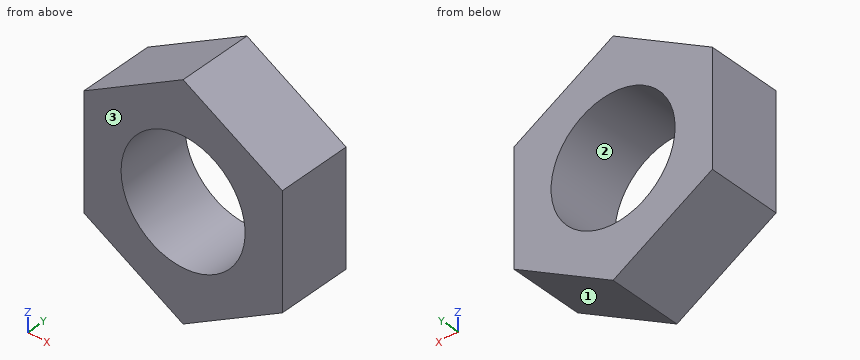
Autodesk Inventor part; units mm, degrees
ref_plane "YZ Plane" through (0, 0, 0) normal (1, 0, 0) x (0, 1, 0)
ref_plane "XZ Plane" through (0, 0, 0) normal (0, 1, 0) x (-1, 0, 0)
ref_plane "XY Plane" through (0, 0, 0) normal (0, 0, 1) x (1, 0, 0)
sketch "Sketch1" plane through (0, 0, 0) normal (0, 1, 0) x (-1, 0, 0)
  line L0 (0, -4.6188) -> (-4, -2.3094)
  line L1 (-4, -2.3094) -> (-4, 2.3094)
  line L2 (-4, 2.3094) -> (0, 4.6188)
  line L3 (0, 4.6188) -> (4, 2.3094)
  line L4 (4, 2.3094) -> (4, -2.3094)
  line L5 (4, -2.3094) -> (0, -4.6188)
  circle A0 centre (0, 0) radius 2.5
  dimension "d0" = 8
  dimension "d1" = 5
extrude "Extrusion1" add sketch "Sketch1" along normal blind 3
thread "Thread1"
properties part number "nut rod"
Could you check a few things on this model? Use its own coordinates, in mm. Face numbers are marked on the shaded views. Coordinates: 2 decimals unless noted, no trailing zeros. Order: outer loops, then holes, each group sorted by start corner. A loop starts at its lowest first (then second) coordinate and runs counter-clockwise, first axis right, second up. Notation, with made-up numbers: M -7,11.25 L 12,11.25 A17 ccw 12,18.25 Z; hole C -8.75,30 d7. An arc over 180 degrees is marked long. Use one line per item in the form item = value. Start each with the question number.
1. For pin 1 (1 mm diameter, centred on x = -2.5, y = 1, fed in from -Z), with a flat end and sliding along its axis, tell me the tip position at first contact or that it passes through.
2. Suppose I cut it at A-A on z = 0. Write out the boundary of the cut face in (x, y), then the cut area to 3 significant figures.
3. We'd pull the mould along Z, two halves only. Please class the marked faces 1, 2 and 3: +Z half, -Z half, draft (parallel to the pull), parting line (faces both ways), or undercut.
4. Suppose I cut it at B-B on y = 1.8. Write out the boundary of the cut face in (x, z).
5. Suppose I cut it at D-D on x = -3. Write out the boundary of the cut face in (y, z).
6. Suppose I cut it at C-C on x = 0.5. Write out the boundary of the cut face in (y, z), then the cut area to 3 significant figures.
7. Please list where these lines run through material, in increasing order: line 1 (X direction, y = 2.6, z = -1); line 2 (X direction, y = 1.9, z = 2.25); line 3 (Z direction, x = 3.75, y = 2.4).
Geometry says:
q1.pin_1 = -3.46
q2.outline = M -4,0 L -2.5,0 L -2.5,3 L -4,3 Z; M 2.5,0 L 4,0 L 4,3 L 2.5,3 Z
q2.area = 9.00 mm^2
q3.face_1 = -Z half
q3.face_2 = undercut
q3.face_3 = draft
q4.outline = M -4,-2.31 L 0,-4.62 L 4,-2.31 L 4,2.31 L 0,4.62 L -4,2.31 Z; hole C 0,0 d5
q5.outline = M 0,-2.89 L 3,-2.89 L 3,2.89 L 0,2.89 Z
q6.outline = M 0,-4.33 L 3,-4.33 L 3,-2.45 L 0,-2.45 Z; M 0,2.45 L 3,2.45 L 3,4.33 L 0,4.33 Z
q6.area = 11.3 mm^2
q7.line_1 = -4 to -2.29, 2.29 to 4
q7.line_2 = -4 to -1.09, 1.09 to 4
q7.line_3 = -2.45 to 2.45
